Input: part model. Units: mm. Frame: model coordinates. Face numbers are marked on the shaded views. Coordinates: 2 decimals unless noted, no trailing zeros. Order: outer loops, then holes, each group sorted by start corner. A loop starts at its lowest first (then second) coordinate and runs counter-clockwise, first axis right, second up. Notation, with made-up numbers: (51, 44) - (76, 44) arc R13 cw to (76, 64) - close; hole circle Ø6 at (-2, 58). An arc over 180 degrees is marked (long way). Use a Markdown table: item, result. Add a question column.
Autodesk Inventor part; units mm, degrees
ref_plane "YZ Plane" through (0, 0, 0) normal (1, 0, 0) x (0, 1, 0)
ref_plane "XZ Plane" through (0, 0, 0) normal (0, 1, 0) x (-1, 0, 0)
ref_plane "XY Plane" through (0, 0, 0) normal (0, 0, 1) x (1, 0, 0)
sketch "Sketch1" plane through (0, 0, 0) normal (1, 0, 0) x (0, 1, 0)
  circle A0 centre (0, -38.1) radius 1.7907
  circle A1 centre (12.7, -12.7) radius 1.7907
  circle A2 centre (25.4, -38.1) radius 1.7907
  line L0 (-12.7, -50.8) -> (38.1, -50.8)
  line L1 (38.1, -25.4) -> (38.1, -50.8)
  line L2 (34.925, -25.4) -> (38.1, -25.4)
  arc A3 (25.4, -15.875) -> (34.925, -25.4) centre (34.925, -15.875) ccw
  line L3 (25.4, -15.875) -> (25.4, 0)
  line L4 (0, 0) -> (25.4, 0)
  line L5 (0, -15.875) -> (0, 0)
  arc A4 (-9.525, -25.4) -> (0, -15.875) centre (-9.525, -15.875) ccw
  line L6 (-9.525, -25.4) -> (-12.7, -25.4)
  line L7 (-12.7, -50.8) -> (-12.7, -25.4)
  point P0 (12.7, -50.8)
extrude "Extrusion1" add sketch "Sketch1" along normal blind 3.2512
sketch "Sketch2" plane through (0, 0, 0) normal (-1, 0, 0) x (0, 0, 1)
  circle A0 centre (-38.1, 25.4) radius 1.7907
  circle A1 centre (-12.7, 12.7) radius 1.7907
  circle A2 centre (-38.1, 0) radius 1.7907
  line L0 (-50.8, -12.7) -> (-50.8, 38.1)
  line L1 (-25.4, -12.7) -> (-50.8, -12.7)
  line L2 (-25.4, -9.525) -> (-25.4, -12.7)
  arc A3 (-15.875, 0) -> (-25.4, -9.525) centre (-15.875, -9.525) ccw
  line L3 (0, 0) -> (-15.875, 0)
  line L4 (0, 25.4) -> (0, 0)
  line L5 (-15.875, 25.4) -> (0, 25.4)
  arc A4 (-25.4, 34.925) -> (-15.875, 25.4) centre (-15.875, 34.925) ccw
  line L6 (-25.4, 38.1) -> (-25.4, 34.925)
  line L7 (-50.8, 38.1) -> (-25.4, 38.1)
  line L8 (0, 25.4) -> (0, 0)
  line L9 (0, 22.225) -> (-28.575, 22.225)
  line L10 (0, 3.175) -> (-28.575, 3.175)
  line L11 (-28.575, 38.1) -> (-28.575, 22.225)
  line L12 (-28.575, 3.175) -> (-28.575, -12.7)
  line L13 (-25.4, -12.7) -> (-50.8, -12.7)
  line L14 (-47.625, 2.0848) -> (-47.625, -12.7)
  line L15 (-47.625, 2.0848) -> (-47.625, 38.1)
  line L16 (-50.8, 38.1) -> (-25.4, 38.1)
  line L17 (-38.1, 38.1) -> (-38.1, 48.6626) construction
  line L18 (-38.1, 52.0515) -> (-28.575, 52.0515) construction
  line L19 (-38.1, 52.0515) -> (-47.625, 52.0515) construction
  line L20 (-38.1, -12.7) -> (-38.1, -13.4551) construction
  line L21 (-38.1, -13.4551) -> (-38.1, -16.9489) construction
  line L22 (-28.575, -16.9489) -> (-38.1, -16.9489) construction
  line L23 (-38.1, -16.9489) -> (-47.625, -16.9489) construction
  line L24 (0, 12.7) -> (-6.3454, 12.7) construction
  line L25 (-3.5322, 12.7) -> (-3.5322, 22.225) construction
  line L26 (-3.5322, 12.7) -> (-3.5322, 3.175) construction
  dimension "d2" = 19.05
  dimension "d3" = 19.05
extrude "Extrusion2" add sketch "Sketch2" along normal blind 1 contours L0 L7 L15 L14 L1 | L12 L10 L4 L3 A3 L2 L1 | L7 L6 A4 L5 L4 L9 L11
properties part number "side holders"
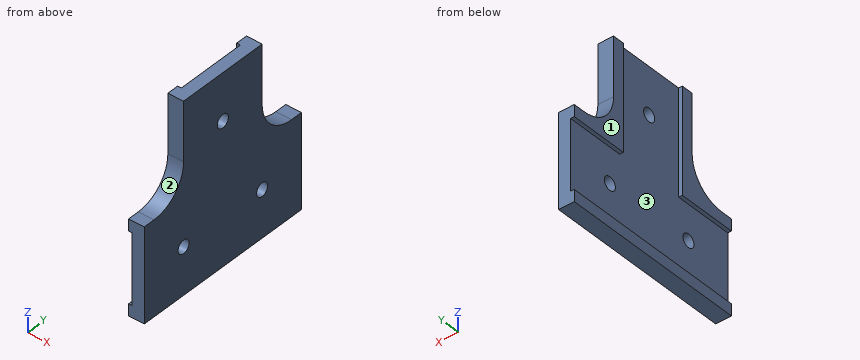
1) Cut plane A-A (x = 1.15). Return the cut outline in (y, z) (3 decimals).
2) Cut plane C-C (y = 12.7). Return the cut outline in (x, z) (3 decimals), and give its area (3 significant figures).
3) Cut plane D-D (z = -12). Return the cut outline in (x, y) (3 decimals), and give its area (3 significant figures).
4) Material intervals for L1, parallel to Z at x = 1.65, y = -9.5; L2, parallel to Z at x = 2.2, y = 12.7; L3, parallel to X at y = 18, z = -25.5, sorted ascending.
5) Cut plane B-B (z = -38.1). Return the cut outline in (x, y), and give its area (3 significant figures).
6) Pull-direction query (Z, two-part tool) for the marked faces 1, 2 and 3; classes: pulls with the +Z half, pulls with the -Z half, needs draft (parallel to the pull), parting line crosses it, or undercut.
7) Contact query for flat-ended pins moving along their axis: P1, Ø0.8, axis at x = -0.5, z = -10, coming from the +Y side; P2, Ø1.5, axis at x = 0.5, z = -6.5, coming from the -Y side; P3, Ø2.5, axis at x = 1.5, y = -11, coming from the +Z side. Output: stop coordinate, or through.
Computed:
| question | item | result |
|---|---|---|
| 1 | outline | (-12.7, -50.8) - (38.1, -50.8) - (38.1, -25.4) - (34.925, -25.4) arc R9.525 cw to (25.4, -15.875) - (25.4, 0) - (0, 0) - (0, -15.875) arc R9.525 cw to (-9.525, -25.4) - (-12.7, -25.4) - close; hole circle Ø3.581 at (0, -38.1); hole circle Ø3.581 at (12.7, -12.7); hole circle Ø3.581 at (25.4, -38.1) |
| 2 | outline | (-1, -50.8) - (3.251, -50.8) - (3.251, -14.491) - (0, -14.491) - (0, -47.625) - (-1, -47.625) - close; (0, -10.909) - (3.251, -10.909) - (3.251, 0) - (0, 0) - close |
| 2 | area | 157 mm2 |
| 3 | outline | (-1, 0) - (3.251, 0) - (3.251, 11.052) - (0, 11.052) - (0, 3.175) - (-1, 3.175) - close; (-1, 22.225) - (0, 22.225) - (0, 14.348) - (3.251, 14.348) - (3.251, 25.4) - (-1, 25.4) - close |
| 3 | area | 78.2 mm2 |
| 4 | L1 | z = -50.8 to -25.4 |
| 4 | L2 | z = -50.8 to -14.49, -10.91 to 0 |
| 4 | L3 | x = 0 to 3.25 |
| 5 | outline | (0, -12.7) - (3.25, -12.7) - (3.25, -1.79) - (0, -1.79) - close; (0, 1.79) - (3.25, 1.79) - (3.25, 23.61) - (0, 23.61) - close; (0, 27.19) - (3.25, 27.19) - (3.25, 38.1) - (0, 38.1) - close |
| 5 | area | 142 mm2 |
| 6 | face 1 | needs draft |
| 6 | face 2 | pulls with the +Z half |
| 6 | face 3 | undercut |
| 7 | P1 | stops at y = 25.4 |
| 7 | P2 | stops at y = 0 |
| 7 | P3 | stops at z = -25.4 |
